Model file for the job. Use its own axes, mm. Give positions to 0.01 mm unless a question says otherwise; leave off trailing zeros. Write each loop counter-clockwise with the first axis right and the second up, starting at its lowest first coordinate (ties: lowest second). Pieces come first, ordered by that corner, then holes.
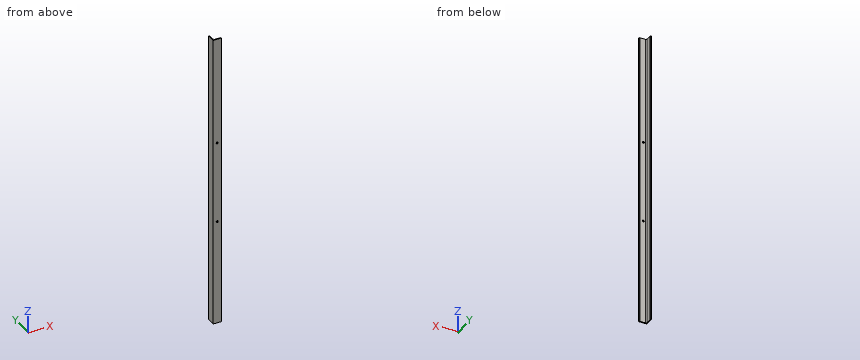
```python
from build123d import *

# Parameters (mm, degrees)
BOSS_EXTRUDE1_DEPTH = 914.4
CUT_EXTRUDE2_REACH  = 52.8
SKETCH5_R           = 6.35


with BuildPart() as part:
    # Sketch1 → Boss-Extrude1 (new body, symmetric)
    with BuildSketch(Plane.XY):
        with BuildLine():
            Line((0, 0), (0, 50.8))
            Line((0, 50.8), (1.59258, 50.8))
            ThreePointArc((1.59258, 50.8), (4.956583943, 49.406583943), (6.35, 46.04258))
            Line((6.35, 46.04258), (6.35, 11.1125))
            ThreePointArc((6.35, 11.1125), (7.744903955, 7.744903955), (11.1125, 6.35))
            Line((11.1125, 6.35), (46.04258, 6.35))
            ThreePointArc((46.04258, 6.35), (49.406583943, 4.956583943), (50.8, 1.59258))
            Line((50.8, 1.59258), (50.8, 0))
            Line((50.8, 0), (0, 0))
        make_face()
    extrude(amount=BOSS_EXTRUDE1_DEPTH, both=True)

    # Sketch5 → Cut-Extrude2 (cut, up to next)
    with BuildSketch(Plane.XZ, mode=Mode.PRIVATE) as cut_extrude2_sk1:
        with Locations((25.4, -261.366)):
            Circle(SKETCH5_R)
    cut_extrude2_tool1 = extrude(cut_extrude2_sk1.sketch, amount=-CUT_EXTRUDE2_REACH, mode=Mode.PRIVATE) & part.part
    add(cut_extrude2_tool1.solids().sort_by_distance((25.4, 0, -261.366))[0], mode=Mode.SUBTRACT)
    # Sketch5 → Cut-Extrude2 (cut, up to next)
    with BuildSketch(Plane.XZ, mode=Mode.PRIVATE) as cut_extrude2_sk2:
        with Locations((25.4, 246.634)):
            Circle(SKETCH5_R)
    cut_extrude2_tool2 = extrude(cut_extrude2_sk2.sketch, amount=-CUT_EXTRUDE2_REACH, mode=Mode.PRIVATE) & part.part
    add(cut_extrude2_tool2.solids().sort_by_distance((25.4, 0, 246.634))[0], mode=Mode.SUBTRACT)


solid = part.part
```
1. Slice it at B-B, the plane y = 36. Write the cut outline in (x, z).
Calculated:
outline: (0, -914.4) - (6.35, -914.4) - (6.35, 914.4) - (0, 914.4) - close
2. Probe probe 1 along Z at (x, y) = (25.4, 3.75); probe 2 along Y at (x, z) = (26.5, -730). List the from-to ranges inside material, lowest first.
Calculated:
probe 1: z = -914.4 to -267.72, -255.02 to 240.28, 252.98 to 914.4
probe 2: y = 0 to 6.35
3. Pin check, flat tips, straight feed: P1, Ø6, axis at y = 17.5, z = 375, coming from the +X side; P2, Ø7.5, axis at x = 25.4, z = 246.634, coming from the -Y side; P3, Ø17.5, axis at x = 32.5, z = 366, coming from the +Y side. Stop position of each tip, or through.
Calculated:
P1: stops at x = 6.35
P2: passes through
P3: stops at y = 6.35
